Autodesk Inventor part; units mm, degrees
ref_plane "YZ Plane" through (0, 0, 0) normal (1, 0, 0) x (0, 1, 0)
ref_plane "XZ Plane" through (0, 0, 0) normal (0, 1, 0) x (-1, 0, 0)
ref_plane "XY Plane" through (0, 0, 0) normal (0, 0, 1) x (1, 0, 0)
sketch "Sketch1" plane through (0, 0, 0) normal (0, 0, 1) x (1, 0, 0)
  line L0 (0, 0) -> (150, 0)
  line L1 (150, 0) -> (150, 164.5751)
  line L2 (150, 164.5751) -> (0, 164.5751)
  line L3 (0, 164.5751) -> (0, 0)
  dimension "d0" = 150
  dimension "d1" = 164.5751
extrude "Extrusion1" add sketch "Sketch1" along normal blind 15
sketch "Sketch7" plane through (0, 0, 0) normal (0, 0, -1) x (-1, 0, 0)
  line L0 (-20, 50) -> (0, 50)
  line L1 (0, 50) -> (0, 100)
  line L2 (0, 100) -> (-20, 100)
  line L3 (-20, 100) -> (-20, 50)
  line L4 (0, 164.5751) -> (0, 0)
  dimension "d27" = 20
  dimension "d28" = 50
  dimension "d96" = 50
extrude "Extrusion7" cut sketch "Sketch7" against normal blind 5
sketch "Sketch8" plane through (0, 0, 0) normal (0, 0, -1) x (-1, 0, 0)
  line L0 (-150, 164.5751) -> (0, 164.5751)
  line L1 (-25, 164.5751) -> (-125, 164.5751)
  line L2 (-125, 164.5751) -> (-125, 184.5751)
  line L3 (-125, 184.5751) -> (-25, 184.5751)
  line L4 (-25, 184.5751) -> (-25, 164.5751)
  point P0 (0, 0)
  dimension "d37" = 100
  dimension "d38" = 20
  dimension "d126" = 25
extrude "Extrusion8" add sketch "Sketch8" against normal blind 5
sketch "Sketch9" plane through (0, 0, 0) normal (0, 0, -1) x (-1, 0, 0)
  circle A0 centre (-50, 174.5751) radius 2.5
  circle A1 centre (-100, 174.5751) radius 2.5
  line L0 (-125, 184.5751) -> (-25, 184.5751)
  line L1 (0, 100) -> (0, 50)
  line L2 (0, 25) -> (20, 25)
  line L3 (20, 75) -> (0, 75)
  point P0 (0, 0)
  dimension "d44" = 5
  dimension "d45" = 5
  dimension "d46" = 10
extrude "Extrusion9" cut sketch "Sketch9" against normal through all
thread "Thread1"
thread "Thread2"
sketch "Sketch12" plane through (0, 0, 0) normal (0, 0, -1) x (-1, 0, 0)
  line L0 (0, 0) -> (-150, 0)
  line L1 (-25, 0) -> (-125, 0)
  line L2 (-125, 0) -> (-125, 20)
  line L3 (-125, 20) -> (-25, 20)
  line L4 (-25, 20) -> (-25, 0)
  dimension "d79" = 100
  dimension "d80" = 20
  dimension "d81" = 25
extrude "Extrusion12" cut sketch "Sketch12" against normal blind 5
sketch "Sketch13" plane through (0, 0, 5) normal (0, 0, -1) x (-1, 0, 0)
  circle A0 centre (-50, 10) radius 2.5
  circle A1 centre (-100, 10) radius 2.5
  line L0 (-25, 20) -> (-25, 0)
  line L1 (-125, 0) -> (-125, 20)
  line L2 (-125, 20) -> (-25, 20)
  point P0 (0, 0)
  dimension "d84" = 5
  dimension "d85" = 5
  dimension "d86" = 25
  dimension "d87" = 25
  dimension "d88" = 10
  dimension "d89" = 10
extrude "Extrusion13" cut sketch "Sketch13" against normal through all
thread "Thread9"
thread "Thread10"
sketch "Sketch14" plane through (0, 0, 5) normal (0, 0, -1) x (-1, 0, 0)
  circle A0 centre (-10, 65) radius 2.5
  circle A1 centre (-10, 85) radius 2.5
  line L0 (-20, 50) -> (-20, 100)
  line L1 (0, 50) -> (-20, 50)
  line L2 (-20, 100) -> (0, 100)
  point P0 (0, 0)
  dimension "d97" = 5
  dimension "d98" = 5
  dimension "d99" = 10
  dimension "d100" = 15
  dimension "d101" = 15
  dimension "d102" = 10
extrude "Extrusion14" cut sketch "Sketch14" against normal through all
thread "Thread11"
thread "Thread12"
sketch "Sketch15" plane through (0, 0, 0) normal (0, 0, -1) x (-1, 0, 0)
  line L0 (-150, 0) -> (-150, 164.5751)
  line L1 (-150, 50) -> (-170, 50)
  line L2 (-170, 50) -> (-170, 100)
  line L3 (-170, 100) -> (-150, 100)
  line L4 (-150, 100) -> (-150, 50)
  point P0 (0, 0)
  dimension "d109" = 20
  dimension "d110" = 50
  dimension "d111" = 50
extrude "Extrusion15" add sketch "Sketch15" against normal blind 5
sketch "Sketch16" plane through (0, 0, 0) normal (0, 0, -1) x (-1, 0, 0)
  circle A0 centre (-160, 65) radius 2.5
  circle A1 centre (-160, 85) radius 2.5
  line L0 (-170, 50) -> (-170, 100)
  line L1 (-150, 50) -> (-170, 50)
  line L2 (-170, 100) -> (-150, 100)
  point P0 (0, 0)
  dimension "d114" = 5
  dimension "d115" = 5
  dimension "d116" = 10
  dimension "d117" = 10
  dimension "d118" = 15
  dimension "d119" = 15
extrude "Extrusion16" cut sketch "Sketch16" against normal through all
thread "Thread13"
thread "Thread14"
sketch "Sketch17" plane through (0, 0, 0) normal (0, 0, -1) x (-1, 0, 0)
  circle A0 centre (-104, 98.5751) radius 2.5
  circle A1 centre (-104, 114.5751) radius 2.5
  line L0 (-150, 0) -> (-150, 50)
  line L1 (-150, 164.5751) -> (0, 164.5751)
  line L2 (0, 164.5751) -> (0, 0)
  dimension "d127" = 5
  dimension "d128" = 5
  dimension "d130" = 16
  dimension "d145" = 50
  dimension "d146" = 104
extrude "Extrusion17" cut sketch "Sketch17" against normal through all
thread "Thread17"
thread "Thread18"
sketch "Sketch18" plane through (0, 0, 0) normal (0, 0, -1) x (-1, 0, 0)
  line L0 (0, 50) -> (0, 0)
  circle A0 centre (0, 25) radius 7.5
  dimension "d142" = 15
extrude "Extrusion18" cut sketch "Sketch18" against normal through all
sketch "Sketch19" plane through (0, 0, 15) normal (0, 0, 1) x (1, 0, 0)
  circle A0 centre (88, 18.5751) radius 2.5
  circle A1 centre (72, 18.5751) radius 2.5
  circle A2 centre (104, 114.5751) radius 2.5
  circle A3 centre (104, 98.5751) radius 2.5
  point P0 (0, 0)
  dimension "d147" = 5
  dimension "d148" = 5
  dimension "d149" = 16
  dimension "d150" = 16
  dimension "d151" = 80
extrude "Extrusion19" cut sketch "Sketch19" against normal blind 5 contours A0 | A1
thread "Thread19"
thread "Thread20"
properties part number "CP007" material "ABS Plastic"
Work out the finished part from the listing and answer in its coordinate system (mm). A direction names the side the tool comes from. Give positions to 0.01 mm unless a question says otherwise; leave off trailing zeros. Loops run counter-clockwise (first coordinate to the right, second up) from the corner with the lowest first, then second, coordinate; pieces in that order, holes last. Notation, with made-up numbers: (5.25, 36) - (26.25, 36) arc R26 ccw to (26.25, 69) - close; hole circle Ø4 at (-16, 58). An arc over 180 degrees is marked (long way). Answer in a Markdown table with one row per item.
(1) For a pull along X with two mould halves and no side action, classify faces 1 (the face through (0, 9, 7)), 2 (the face through (10, 100, 2)), 3 (the face through (72, 19, 10)) as pulls with the +X half, pulls with the -X half, needs draft (parallel to the pull), parting line crosses it, or undercut.
Results list:
| item | result |
|---|---|
| face 1 | pulls with the -X half |
| face 2 | needs draft |
| face 3 | undercut |
(2) A tool of negligible diameter and unlimited length cuts with its end or side. For faces 4 (the face through (88, 19, 10)), 5 (the face through (25, 10, 2)), 6 (the face through (25, 175, 2)), 7 (the face through (20, 75, 2)), from which of +Z, -Z, +X, -X, +Y, -Y can it reach the whole face along a straight path? Write none if from no direction.
Results list:
| item | result |
|---|---|
| face 4 | +Z |
| face 5 | -Z, -Y |
| face 6 | +Z, -Z, -X, +Y |
| face 7 | -Z, -X |
(3) Section B-B (y = 10) is taken. Give the vertices of the cut face in (x, z), and give its area (3 significant figures).
Results list:
| item | result |
|---|---|
| outline | (0, 0) - (25, 0) - (25, 5) - (47.5, 5) - (47.5, 15) - (0, 15) - close; (52.5, 5) - (97.5, 5) - (97.5, 15) - (52.5, 15) - close; (102.5, 5) - (125, 5) - (125, 0) - (150, 0) - (150, 15) - (102.5, 15) - close |
| area | 1,650 mm² |
(4) Consider L1, parallel to Y at x = 104, z = 8.75; L2, parallel to Y at x = 104, z = 4.75; L3, parallel to Y at x = 50, z = 11.5. Determine where each line is inside the solid, lowest interval first. Write a range as [from, to].
Results list:
| item | result |
|---|---|
| L1 | y = [0, 96.08], [101.08, 112.08], [117.08, 164.58] |
| L2 | y = [20, 96.08], [101.08, 112.08], [117.08, 184.58] |
| L3 | y = [0, 7.5], [12.5, 164.58] |
(5) Section A-A (x = 10) is taken. Give the vertices of the cut face in (y, z).
Results list:
| item | result |
|---|---|
| outline | (0, 0) - (50, 0) - (50, 5) - (62.5, 5) - (62.5, 15) - (0, 15) - close; (67.5, 5) - (82.5, 5) - (82.5, 15) - (67.5, 15) - close; (87.5, 5) - (100, 5) - (100, 0) - (164.58, 0) - (164.58, 15) - (87.5, 15) - close |
(6) Section C-C (x = 109) is taken. Give the vertices of the cut face in (y, z).
Results list:
| item | result |
|---|---|
| outline | (0, 5) - (20, 5) - (20, 0) - (184.58, 0) - (184.58, 5) - (164.58, 5) - (164.58, 15) - (0, 15) - close |
(7) Section D-D (z = 7.5) is taken. Give the vertices of the cut face in (x, y), and give its area (3 significant figures).
Results list:
| item | result |
|---|---|
| outline | (0, 0) - (150, 0) - (150, 164.58) - (0, 164.58) - (0, 32.5) arc R7.5 cw to (0, 17.5) - close; hole circle Ø5 at (10, 65); hole circle Ø5 at (10, 85); hole circle Ø5 at (50, 10); hole circle Ø5 at (100, 10); hole circle Ø5 at (104, 98.58); hole circle Ø5 at (104, 114.58) |
| area | 24,500 mm² |
(8) Flat-ended cylindrical pins translate along their axes: pin 1 Ø4.5 at (y, z) = (94.5, 8.5) entering from +X; pin 2 Ø2 at (x, z) = (40, 12) entering from +Y; pin 3 Ø4 at (y, z) = (79, 2) entering from -X. Find the tip coordinate at first contact, or state that the pin passes through.
Results list:
| item | result |
|---|---|
| pin 1 | stops at x = 150 |
| pin 2 | stops at y = 164.58 |
| pin 3 | stops at x = 20 |
